Read the model definition and answer for the solid it produces. Units are mm, in the model's axes. A direction names the side the tool comes from. Give positions to 0.01 mm unless a question says otherwise; leave off trailing zeros. Write each loop counter-clockwise with the first axis right and the second up, starting at its lowest first coordinate (ties: lowest second). Pieces come first, ordered by that corner, then holes. Notation, with made-up numbers: M 47,32 L 59,32 A23 ccw 59,46 Z; hole C 8.25,11.25 d6. An arc over 180 degrees is marked long. Put each result on its own line as item: value.
from build123d import *

# Parameters (mm, degrees)
SKETCH1_W           = 40
SKETCH1_H           = 20
BOSS_EXTRUDE1_DEPTH = 6
SKETCH2_W           = 22
SKETCH2_H           = 7
CUT_EXTRUDE1_DEPTH  = 1.2
SKETCH4_R           = 1.5
CUT_EXTRUDE2_DEPTH  = 2.8
CUT_EXTRUDE2_TAPER  = 23
SKETCH5_R           = 0.3
CUT_EXTRUDE3_DEPTH  = 2.5


with BuildPart() as part:
    # Sketch1 → Boss-Extrude1 (new body)
    with BuildSketch(Plane.XY):
        Rectangle(SKETCH1_W, SKETCH1_H)
    extrude(amount=BOSS_EXTRUDE1_DEPTH)

    # Sketch2 → Cut-Extrude1 (cut)
    with BuildSketch(Plane.XY.offset(6)):
        Rectangle(SKETCH2_W, SKETCH2_H)
    extrude(amount=-CUT_EXTRUDE1_DEPTH, mode=Mode.SUBTRACT)

    # Sketch4 → Cut-Extrude2 (cut)
    with BuildSketch(Plane.XY.offset(4.8)):
        with Locations((-7.72, 0)):
            Circle(SKETCH4_R)
        with Locations((-3.8, 0)):
            Circle(SKETCH4_R)
        with Locations((3.8, 0)):
            Circle(SKETCH4_R)
        with Locations((7.72, 0)):
            Circle(SKETCH4_R)
    extrude(amount=-CUT_EXTRUDE2_DEPTH, taper=CUT_EXTRUDE2_TAPER, mode=Mode.SUBTRACT)

    # Sketch5 → Cut-Extrude3 (cut)
    with BuildSketch(Plane.XY.offset(2)):
        with Locations((-7.72, 0)):
            Circle(SKETCH5_R)
        with Locations((-3.8, 0)):
            Circle(SKETCH5_R)
        with Locations((3.8, 0)):
            Circle(SKETCH5_R)
        with Locations((7.72, 0)):
            Circle(SKETCH5_R)
    extrude(amount=-CUT_EXTRUDE3_DEPTH, mode=Mode.SUBTRACT)


solid = part.part
(1) Straight lines are drawn through the part: line 1 along Y through (x, z) = (-3.8, 0.7); line 2 along Z through (x, y) = (-0.5, -0.75); line 3 along Y through (x, z) = (-5.5, 5.2). For each, find the intervals that lie inside material, in ascending order. Write a range as from..to.
Result:
line 1: y = -10..-0.3, 0.3..10
line 2: z = 0..4.8
line 3: y = -10..-3.5, 3.5..10
(2) Which of the six approach directions +Z, -Z, +X, -X, +Y, -Y give full straight-line access (tool end or side, diameter ignored) to faces 4 (the face through (0, 10, 3)), 5 (the face through (0, 3.5, 5))?
Result:
face 4: +Z, -Z, +X, -X, +Y
face 5: +Z
(3) Given pin 1 Ø1.5 at (x, y) = (7.5, 0.5) entering from +Z; pin 2 Ø0.7 at (x, y) = (-3.5, 0) entering from +Z; pin 3 Ø0.5 at (x, y) = (8, 0) entering from +Z, each flat-ended and moving along its own axis, determine where each tip first touches the part or whether it passes through.
Result:
pin 1: stops at z = 4.32
pin 2: stops at z = 2.8
pin 3: stops at z = 2.51
(4) Section A-A on x = 0.5 is taken. Determine the outline of the cut face in (y, z), and give its area (3 significant figures).
Result:
outline: M -10,0 L 10,0 L 10,6 L 3.5,6 L 3.5,4.8 L -3.5,4.8 L -3.5,6 L -10,6 Z
area: 112 mm²
(5) For a pull along Y with two mould halves and no side action, classify faces 1 (the face through (11, 0, 5)), 2 (the face through (20, 0, 3)), 3 (the face through (0, -10, 3)) as +Y half, -Y half, draft (parallel to the pull), parting line (faces both ways), or undercut.
Result:
face 1: undercut
face 2: draft
face 3: -Y half
(6) Section B-B on y = -2.5 is taken. Determine the outline of the cut face in (x, z).
Result:
outline: M -20,0 L 20,0 L 20,6 L 11,6 L 11,4.8 L -11,4.8 L -11,6 L -20,6 Z
